from build123d import *

# Parameters (mm, degrees)
SKETCH1_W               = 85
SKETCH1_H               = 200
BOSS_EXTRUDE1_DEPTH     = 5
FILLET1_R               = 1
SKETCH2_R               = 17.5
CUT_EXTRUDE1_DEPTH      = 2.5
FILLET2_R               = 0.125
SKETCH3_W               = 15
SKETCH3_H               = 85
BOSS_EXTRUDE2_DEPTH     = 3
RIB1_START              = -5
RIB1_DEPTH              = 5
SKETCH5_R               = 1.5
CUT_EXTRUDE2_DEPTH      = 3
FILLET3_R               = 4
FILLET4_R               = 3
SKETCH6_OUTSIDE_W       = 130.646
SKETCH6_OUTSIDE_H       = 245.646
SKETCH6_OUTSIDE_R       = 17.5
CUT_EXTRUDE4_DEPTH      = 206.441597541
CUT_EXTRUDE5_DEPTH      = 194.642389471
CUT_EXTRUDE5_DEPTH_BACK = 194.642389471
CUT_EXTRUDE6_START      = -1.5
SKETCH9_R               = 17.5
CUT_EXTRUDE6_DEPTH      = 1.5


# Read off the part's stored shape, not the designer's step: Rib1
with BuildPart() as part:
    # Sketch1 → Boss-Extrude1 (new body)
    with BuildSketch(Plane(origin=(0, 0, 0), x_dir=(0, 0, -1), z_dir=(1, 0, 0))):
        with Locations((0, 100)):
            Rectangle(SKETCH1_W, SKETCH1_H)
        Polygon((-16, 25), (-16, 176), (-11, 176), (-11, 49), (-7, 49), (-7, 29), (-2.5, 29), (-2.5, 42), (16, 42), (16, 25), (16, 24), (15, 24), (-15, 24), (-16, 24), align=None, mode=Mode.SUBTRACT)
    extrude(amount=BOSS_EXTRUDE1_DEPTH)

    # Fillet1
    fillet1_edges = [part.edges().sort_by_distance(p)[0] for p in [
        (2.5, 42, 2.5),
        (2.5, 29, 2.5),
        (2.5, 29, 7),
        (2.5, 49, 11),
    ]]
    fillet(fillet1_edges, radius=FILLET1_R)

    # Sketch2 → Cut-Extrude1 (cut)
    with BuildSketch(Plane(origin=(5, 0, 0), x_dir=(0, 0, -1), z_dir=(1, 0, 0))):
        with Locations((15.75, 173.25)):
            Circle(SKETCH2_R)
        Polygon((15.75, 173.125), (15.625, 173.25), (8.75, 173.25), (15.75, 187.25), (15.75, 173.375), (15.875, 173.25), (22.75, 173.25), (15.75, 159.25), align=None, mode=Mode.SUBTRACT)
    extrude(amount=-CUT_EXTRUDE1_DEPTH, mode=Mode.SUBTRACT)

    # Fillet2
    fillet2_edges = [part.edges().sort_by_distance(p)[0] for p in [
        (3.75, 173.25, -15.625),
        (3.75, 173.125, -15.75),
        (3.75, 173.25, -15.875),
        (3.75, 173.375, -15.75),
    ]]
    fillet(fillet2_edges, radius=FILLET2_R)

    # Sketch3 → Boss-Extrude2 (add)
    with BuildSketch(Plane.XZ):
        with Locations((-7.5, 0)):
            Rectangle(SKETCH3_W, SKETCH3_H)
    extrude(amount=-BOSS_EXTRUDE2_DEPTH)

    # Rib1 outline → Rib1 (add)
    with BuildSketch(Plane.XY.offset(42.5).offset(RIB1_START)):
        Polygon((0, 18), (-15, 3), (0, 3), align=None)
    rib1 = extrude(amount=RIB1_DEPTH)

    # Mirror1: Rib1 across plane
    add(rib1.mirror(Plane.XY))

    # Sketch5 → Cut-Extrude2 (cut)
    with BuildSketch(Plane(origin=(0, 3, 0), x_dir=(1, 0, 0), z_dir=(0, 1, 0))):
        with Locations(Location((-7.5, 24.5, 0), (0, 0, 270))):
            Circle(SKETCH5_R)
        with Locations(Location((-7.5, 0, 0), (0, 0, 270))):
            Circle(SKETCH5_R)
        with Locations(Location((-7.5, -24.5, 0), (0, 0, 270))):
            Circle(SKETCH5_R)
    extrude(amount=-CUT_EXTRUDE2_DEPTH, mode=Mode.SUBTRACT)

    # Fillet3
    fillet3_edges = [part.edges().sort_by_distance(p)[0] for p in [
        (0, 18, 40),
        (0, 18, -40),
    ]]
    fillet(fillet3_edges, radius=FILLET3_R)

    # Fillet4
    fillet4_edges = [part.edges().sort_by_distance(p)[0] for p in [
        (0, 3, 0),
    ]]
    fillet(fillet4_edges, radius=FILLET4_R)

    # Sketch6 outside → Cut-Extrude4 (cut, through all)
    with BuildSketch(Plane(origin=(5, 0, 0), x_dir=(0, 0, -1), z_dir=(1, 0, 0))):
        with Locations((0, 100)):
            Rectangle(SKETCH6_OUTSIDE_W, SKETCH6_OUTSIDE_H)
        with Locations((15.75, 173.25)):
            Circle(SKETCH6_OUTSIDE_R, mode=Mode.SUBTRACT)
    extrude(amount=-CUT_EXTRUDE4_DEPTH, mode=Mode.SUBTRACT)

    # Sketch7 → Cut-Extrude5 (cut, two sides: drawn at the far end of the back side and taken through both)
    with BuildSketch(Plane(origin=(2.5, 0, 0), x_dir=(0, 0, -1), z_dir=(1, 0, 0)).offset(-CUT_EXTRUDE5_DEPTH_BACK)):
        with BuildLine():
            Line((22.75, 173.25), (15.75, 159.25))
            Line((15.75, 159.25), (15.75, 173.073223305))
            ThreePointArc((15.75, 173.073223305), (15.740484942, 173.121058734), (15.713388348, 173.161611652))
            Line((15.713388348, 173.161611652), (15.661611652, 173.213388348))
            ThreePointArc((15.661611652, 173.213388348), (15.621058734, 173.240484942), (15.573223305, 173.25))
            Line((15.573223305, 173.25), (8.75, 173.25))
            Line((8.75, 173.25), (15.75, 187.25))
            Line((15.75, 187.25), (15.75, 173.426776695))
            ThreePointArc((15.75, 173.426776695), (15.759515058, 173.378941266), (15.786611652, 173.338388348))
            Line((15.786611652, 173.338388348), (15.838388348, 173.286611652))
            ThreePointArc((15.838388348, 173.286611652), (15.878941266, 173.259515058), (15.926776695, 173.25))
            Line((15.926776695, 173.25), (22.75, 173.25))
        make_face()
    extrude(amount=CUT_EXTRUDE5_DEPTH + CUT_EXTRUDE5_DEPTH_BACK, mode=Mode.SUBTRACT)

    # Sketch9 → Cut-Extrude6 (cut)
    with BuildSketch(Plane.ZY.offset(CUT_EXTRUDE6_START)):
        with Locations(Location((-15.75, 173.25, 0), (0, 0, 180))):
            Circle(SKETCH9_R)
    extrude(amount=CUT_EXTRUDE6_DEPTH, mode=Mode.SUBTRACT)


solid = part.part
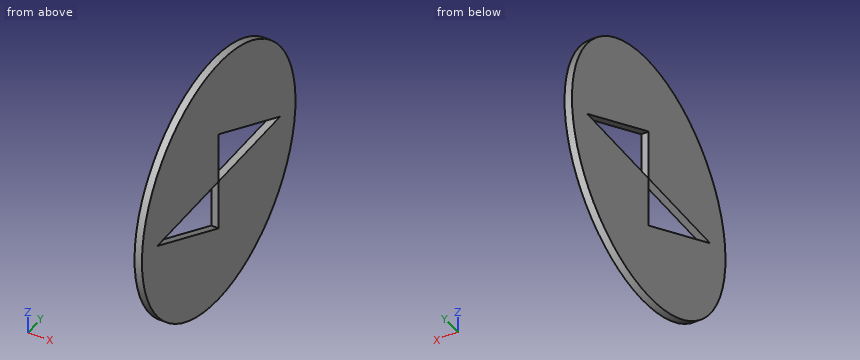
Could you check a few things on this model? Use its own coordinates, in mm. Give positions to 0.01 mm unless a question says otherwise; leave off trailing zeros. Order: outer loops, then holes, each group sorted by start corner. A loop starts at its lowest first (then second) coordinate and runs counter-clockwise, first axis right, second up. Notation, with made-up numbers: (-4, -21) - (30, -21) arc R21 ccw to (30, 4) - close; hole circle Ø8 at (2.5, 3.25). An arc over 180 degrees is marked (long way). Return JSON: item names as keys, results as strings. Group by question number.
Q1. Suppose I cut it at B-B, the plane y = 181. Please give me the cut outline in (x, z) (3 decimals), and give its area (3 significant figures).
Q2. Suppose I cut it at C-C, the plane z = -19. Please give me the cut outline in (x, y), and give its area (3 significant figures).
Q3. Please list where these lines run through material, in increasing order: line 1 along Z through (x, y) = (1.6, 183) (3 decimals); line 2 along Y through (x, z) = (2, -22.5); line 3 along Z through (x, y) = (1.7, 166) (3 decimals). Write a range as [from, to].
Q4. Will this pin go through, and if not, where does the flat tip stop? pin 1 Ø0.5 at (x, y) = (2, 178.5) entering from +Z.
Q5. Suppose I cut it at D-D, the plane z = -29. Please give me the cut outline in (x, y), and give its area (3 significant figures).
Q6. Suppose I cut it at A-A, the plane x = 1.7. Please give me the cut outline in (y, z) (3 decimals).
Resolved:
{
 "1": {"outline": "(1.5, -31.44) - (2.5, -31.44) - (2.5, -15.75) - (1.5, -15.75) - close; (1.5, -12.625) - (2.5, -12.625) - (2.5, -0.06) - (1.5, -0.06) - close", "area": "28.3 mm2"},
 "2": {"outline": "(1.5, 156.05) - (2.5, 156.05) - (2.5, 165.75) - (1.5, 165.75) - close; (1.5, 173.25) - (2.5, 173.25) - (2.5, 190.45) - (1.5, 190.45) - close", "area": "26.9 mm2"},
 "3": {"line 1": "z = [-30.282, -15.75], [-13.625, -1.218]", "line 2": "y = [157.1, 172.75], [173.25, 189.4]", "line 3": "z = [-31.678, -19.125], [-15.75, 0.178]"},
 "4": {"pin 1": "stops at z = 1.02"},
 "5": {"outline": "(1.5, 161.82) - (2.5, 161.82) - (2.5, 184.68) - (1.5, 184.68) - close", "area": "22.9 mm2"},
 "6": {"outline": "circle Ø35 at (173.25, -15.75); hole (159.25, -15.75) - (173.25, -22.75) - (173.25, -15.927) arc R0.125 cw to (173.287, -15.838) - (173.338, -15.787) arc R0.125 cw to (173.427, -15.75) - (187.25, -15.75) - (173.25, -8.75) - (173.25, -15.573) arc R0.125 cw to (173.213, -15.662) - (173.162, -15.713) arc R0.125 cw to (173.073, -15.75) - close"}
}
